For this review, use the dimensioned drawing (mm, ordinates from the lowest corner) and the shaded views. Round coordinates to 2 decimals unless told otherwise and drop trailing zeros. Loops run counter-clockwise (first coordinate to the right, second up) from the corner with the lowest first, then second, coordinate; pieces in that order, holes last. Notation, with made-up numbers: M 32,45.5 L 83,45.5 A32 ccw 83,83.5 Z; hole C 38,18 d4. An arc over 180 degrees is marked long. Answer as a JSON object with one key per item and string values. Group by question number.
Item 1: Insertion check: P1, Ø1, axis at x = 11.5, z = 75.5, coming from the -Y side; P2, Ø1.5, axis at x = 14.5, z = 47, coming from the +Y side; P3, Ø4, axis at y = 13, z = 26, coming from the -X side. Each pin has a flat end and moves straight along its axis. Give the tip position at first contact, or say it passes through.
Item 2: Consider section D-D (x = 17.75). Give the boundary of the cut face in (y, z) (1 decimal).
Item 3: Consider section B-B (x = 3.5). Give the boundary of the cut face in (y, z) (1 decimal).
Item 4: To check wall thickness, follow line 1 (Y direction, x = 9, z = 77); line 2 (X direction, y = 7.5, z = 68) (1 decimal); line 3 (Y direction, x = 15.5, z = 59) (1 decimal). State the ranges of each line that lie inside material, in increasing order.
Item 5: Consider section A-A (y = 11). Give the boundary of the cut face in (x, z) (1 decimal).
Item 6: Consider section C-C (z = 69). Give the boundary of the cut face in (x, y) (1 decimal).
Item 7: The part is to be moulded in two halves that separate along X. For the marked faces 1 and 2, say which applies: +X half, -X half, draft (parallel to the pull), parting line (faces both ways), or undercut.
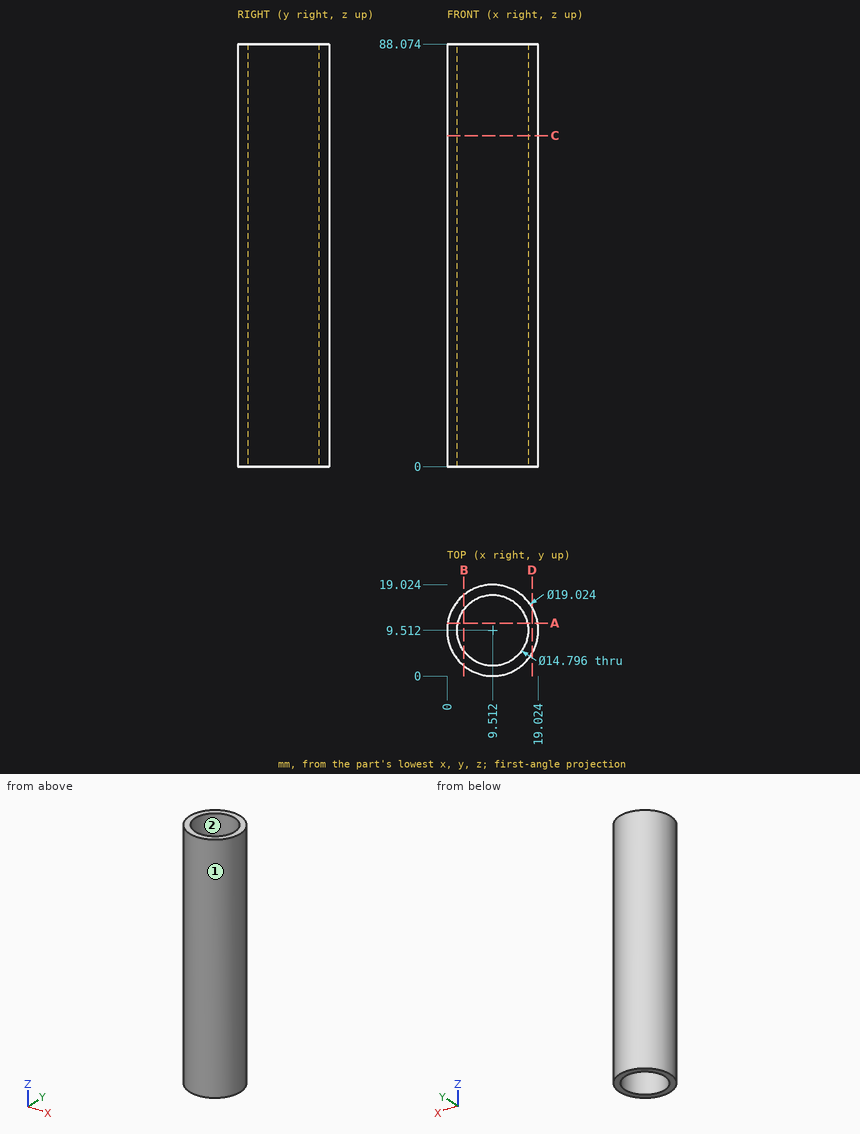
Geometry results:
{
 "1": {"P1": "stops at y = 0.12", "P2": "stops at y = 18.03", "P3": "stops at x = 0.12"},
 "2": {"outline": "M 4.8,0 L 14.3,0 L 14.3,88.1 L 4.8,88.1 Z"},
 "3": {"outline": "M 2.1,0 L 5.2,0 L 5.2,88.1 L 2.1,88.1 Z; M 13.8,0 L 16.9,0 L 16.9,88.1 L 13.8,88.1 Z"},
 "4": {"line 1": "y = 0.01 to 2.13, 16.89 to 19.01", "line 2": "x = 0.2 to 2.4, 16.6 to 18.8", "line 3": "y = 2.1 to 5.2, 13.9 to 16.9"},
 "5": {"outline": "M 0.1,0 L 2.3,0 L 2.3,88.1 L 0.1,88.1 Z; M 16.8,0 L 18.9,0 L 18.9,88.1 L 16.8,88.1 Z"},
 "6": {"outline": "C 9.5,9.5 d19; hole C 9.5,9.5 d14.8"},
 "7": {"face 1": "parting line", "face 2": "undercut"}
}
